```python
from build123d import *

# Parameters (mm, degrees)
SKETCH1_W           = 20
SKETCH1_H           = 20
SKETCH1_W_2         = 17
SKETCH1_H_2         = 17
BOSS_EXTRUDE1_DEPTH = 200
SKETCH2_R           = 2.125
CUT_EXTRUDE1_DEPTH  = 202.246117975


with BuildPart() as part:
    # Sketch1 → Boss-Extrude1 (new body)
    with BuildSketch(Plane.XY):
        Rectangle(SKETCH1_W, SKETCH1_H)
        Rectangle(SKETCH1_W_2, SKETCH1_H_2, mode=Mode.SUBTRACT)
    extrude(amount=-BOSS_EXTRUDE1_DEPTH)

    # Sketch2 → Cut-Extrude1 (cut, through all)
    with BuildSketch(Plane(origin=(0, 10, 0), x_dir=(1, 0, 0), z_dir=(0, 1, 0))):
        with Locations(Location((0, 10, 0), (0, 0, 270))):
            Circle(SKETCH2_R)
        with Locations(Location((0, 70, 0), (0, 0, 270))):
            Circle(SKETCH2_R)
        with Locations(Location((0, 130, 0), (0, 0, 270))):
            Circle(SKETCH2_R)
        with Locations(Location((0, 190, 0), (0, 0, 270))):
            Circle(SKETCH2_R)
    extrude(amount=-CUT_EXTRUDE1_DEPTH, mode=Mode.SUBTRACT)


solid = part.part
```
For this review, take the finished solid that the model builds, in its own axes (mm). A direction names the side the tool comes from. Round coordinates to 2 decimals unless told otherwise and drop trailing zeros. Order: outer loops, then holes, each group sorted by start corner. A loop starts at its lowest first (then second) coordinate and runs counter-clockwise, first axis right, second up. Notation, with made-up numbers: (75, 21) -> (102, 21) arc R16 cw to (102, 26) -> close; hole circle Ø10 at (25.5, 39.25). An arc over 180 degrees is marked (long way). Use a Markdown table: item, result.
Item 1: Draft analysis for pull direction Z (two halves, no side actions). For faces 1 (the flat face through (0, 10, -99)), 2 (the flat face through (-9, 0, -200)), 3 (the cylindrical face through (2.107, -9.24, -10.277)), 4 (the cylindrical face through (0.093, 9.26, -132.123)), state which applies: +Z half, -Z half, draft (parallel to the pull), parting line (faces both ways), or undercut.
Resolved:
| item | result |
|---|---|
| face 1 | draft |
| face 2 | -Z half |
| face 3 | undercut |
| face 4 | undercut |
Item 2: For pin 1 (5 mm diameter, centred on x = 0, z = -70, fed in from -Y), flat-tipped, find the tip position at first contact; note if it passes through.
Resolved:
| item | result |
|---|---|
| pin 1 | stops at y = -10 |
Item 3: Take a section at B-B (y = 1). State the section outline as (x, z) points.
Resolved:
| item | result |
|---|---|
| outline | (-10, -200) -> (-8.5, -200) -> (-8.5, 0) -> (-10, 0) -> close; (8.5, -200) -> (10, -200) -> (10, 0) -> (8.5, 0) -> close |
Item 4: For line 1 along X through (y, z) = (9.15, -130) (3 decimals); line 2 along Y through (x, z) = (5.25, -147), list the stretches that pass through material, from the lowest coordinate up. Write a range as [from, to].
Resolved:
| item | result |
|---|---|
| line 1 | x = [-10, -2.125], [2.125, 10] |
| line 2 | y = [-10, -8.5], [8.5, 10] |
Item 5: Machinability: for faces 5 (the flat face through (0, -10, -99)), 6 (the flat face through (-8.5, 0, -99)), which of the approach directions +Z, -Z, +X, -X, +Y, -Y give a long, thin tool a straight path to every point of the face, cutting with its end or side? Answer none if there is none.
Resolved:
| item | result |
|---|---|
| face 5 | +Z, -Z, +X, -X, -Y |
| face 6 | +Z, -Z |
Item 6: Take a section at C-C (z = -96). State the section outline as (x, y) points.
Resolved:
| item | result |
|---|---|
| outline | (-10, -10) -> (10, -10) -> (10, 10) -> (-10, 10) -> close; hole (-8.5, -8.5) -> (8.5, -8.5) -> (8.5, 8.5) -> (-8.5, 8.5) -> close |
Item 7: Take a section at A-A (z = -70). State the section outline as (x, y) points (3 decimals), plus the area to 4 significant figures.
Resolved:
| item | result |
|---|---|
| outline | (-10, -10) -> (-2.125, -10) -> (-2.125, -8.5) -> (-8.5, -8.5) -> (-8.5, 8.5) -> (-2.125, 8.5) -> (-2.125, 10) -> (-10, 10) -> close; (2.125, -10) -> (10, -10) -> (10, 10) -> (2.125, 10) -> (2.125, 8.5) -> (8.5, 8.5) -> (8.5, -8.5) -> (2.125, -8.5) -> close |
| area | 98.25 mm² |
